from build123d import *

# Parameters (mm, degrees)
SKETCH_1_R      = 2
EXTRUDE_1_DEPTH = 3
EXTRUDE_2_DEPTH = 3
RIB_6_REACH     = 175.393
SKETCH_4_WALL_W = 365.010042788
SKETCH_4_WALL_H = 3
RIB_7_REACH     = 175.393
SKETCH_5_WALL_W = 365.010042788
SKETCH_5_WALL_H = 3
FILLET_1_R      = 2


with BuildPart() as part:
    # Эскиз1 → Бобышка-Вытянуть1 (new body)
    with BuildSketch(Plane(origin=(0, 0, 0), x_dir=(0, 0, -1), z_dir=(1, 0, 0))):
        with BuildLine():
            Line((0, 3), (0, 83))
            ThreePointArc((0, 83), (0.878679656, 85.121320344), (3, 86))
            Line((3, 86), (147, 86))
            ThreePointArc((147, 86), (149.121320344, 85.121320344), (150, 83))
            Line((150, 83), (150, 3))
            ThreePointArc((150, 3), (149.121320344, 0.878679656), (147, 0))
            Line((147, 0), (3, 0))
            ThreePointArc((3, 0), (0.878679656, 0.878679656), (0, 3))
        make_face()
        with Locations((6, 80)):
            Circle(SKETCH_1_R, mode=Mode.SUBTRACT)
        with Locations((144, 80)):
            Circle(SKETCH_1_R, mode=Mode.SUBTRACT)
        with Locations((120, 6)):
            Circle(SKETCH_1_R, mode=Mode.SUBTRACT)
        with Locations((6, 16)):
            Circle(SKETCH_1_R, mode=Mode.SUBTRACT)
        with BuildLine():
            Line((9, 74.803847577), (9, 21.196152423))
            ThreePointArc((9, 21.196152423), (11.196152423, 19), (12, 16))
            Line((12, 16), (12, 12))
            ThreePointArc((12, 12), (12.878679656, 9.878679656), (15, 9))
            Line((15, 9), (114.803847577, 9))
            ThreePointArc((114.803847577, 9), (120, 12), (125.196152423, 9))
            Line((125.196152423, 9), (138, 9))
            ThreePointArc((138, 9), (140.121320344, 9.878679656), (141, 12))
            Line((141, 12), (141, 74.803847577))
            ThreePointArc((141, 74.803847577), (139.757359313, 75.757359313), (138.803847577, 77))
            Line((138.803847577, 77), (11.196152423, 77))
            ThreePointArc((11.196152423, 77), (10.242640687, 75.757359313), (9, 74.803847577))
        make_face(mode=Mode.SUBTRACT)
    extrude(amount=EXTRUDE_1_DEPTH)

    # Эскиз2 → Бобышка-Вытянуть2 (add)
    with BuildSketch(Plane(origin=(0, 0, -50), x_dir=(-1, 0, 0), z_dir=(0, 0, -1))):
        with BuildLine():
            Line((0, 86), (-13, 86))
            Line((-13, 86), (-13, 68))
            Line((-13, 68), (-6, 68))
            ThreePointArc((-6, 68), (-4, 66), (-6, 64))
            Line((-6, 64), (-13, 64))
            Line((-13, 64), (-13, 22))
            Line((-13, 22), (-6, 22))
            ThreePointArc((-6, 22), (-4, 20), (-6, 18))
            Line((-6, 18), (-13, 18))
            Line((-13, 18), (-13, 0))
            Line((-13, 0), (0, 0))
            Line((0, 0), (0, 86))
        make_face()
    extrude(amount=EXTRUDE_2_DEPTH)

    # Эскиз4 wall → Ребро6 (add, up to next)
    with BuildSketch(Plane(origin=(7.056201664, 86, -60.025547367), x_dir=(-0.499999999996, 0, -0.866025403787), z_dir=(-0.866025403787, 0, 0.499999999996)), mode=Mode.PRIVATE) as rib_6_sk1:
        with Locations((0, 1.5)):
            Rectangle(SKETCH_4_WALL_W, SKETCH_4_WALL_H)
    rib_6_tool1 = extrude(rib_6_sk1.sketch, amount=RIB_6_REACH, mode=Mode.PRIVATE) - part.part
    add(rib_6_tool1.solids().sort_by_distance((7.056201664, 86, -60.025547367))[0])

    # Эскиз5 wall → Ребро7 (add, up to next)
    with BuildSketch(Plane(origin=(7.056201664, 0, -60.025547367), x_dir=(-0.499999999996, 0, -0.866025403787), z_dir=(0.866025403787, 0, -0.499999999996)), mode=Mode.PRIVATE) as rib_7_sk1:
        with Locations((0, 1.5)):
            Rectangle(SKETCH_5_WALL_W, SKETCH_5_WALL_H)
    rib_7_tool1 = extrude(rib_7_sk1.sketch, amount=-RIB_7_REACH, mode=Mode.PRIVATE) - part.part
    add(rib_7_tool1.solids().sort_by_distance((7.056201664, 0, -60.025547367))[0])

    # Скругление1
    fillet_1_edges = [part.edges().sort_by_distance(p)[0] for p in [
        (1.5, 77, -50),
        (1.5, 77, -53),
        (1.5, 9, -50),
        (1.5, 9, -53),
    ]]
    fillet(fillet_1_edges, radius=FILLET_1_R)


solid = part.part
Build history of the part. All positions in model axes, mm. A direction names the side the tool comes from. Coordinates: 2 decimals unless noted, no trailing zeros. Write each loop counter-clockwise with the first axis right and the second up, starting at its lowest first coordinate (ties: lowest second). Pieces come first, ordered by that corner, then holes.
(1) Cut at D-D on x = 9.5. List the corners of the cut face in (y, z).
(2) Mould opens along Z. For faces 1 (the flat face through (7.11, 84.48, -59.93)), 2 (the flat face through (9, 18, -51)), 3 (the flat face through (1, 9, -31)) say: pulls with the +Z half, pulls with the -Z half, needs draft (parallel to the pull), parting line crosses it, or undercut.
(3) Cut at A-A on y = 60.5. List the corners of the cut face in (x, z).
(4) Cut at C-C on y = 6. List the corners of the cut face in (x, z).
(5) 3-axis set-ups, long thin cutter, end or side, ignore diameter. For faces 4 (the flat face through (2, 0, -75)), 5 (the flat face through (7, 44, -53)), 6 (the flat face through (1, 9, -132)), 7 (the flat face through (10, 22, -51)), 8 (the flat face through (6, 3, -57)): which of +Z, -Z, +X, -X, +Y, -Y reach the whole face in a straight line?
(6) Cut at B-B on z = -99. List the corners of the cut face in (x, y).
(7) Drill centre lines: line 1 (Y direction, x = 1.25, z = -6); line 2 (Y direction, x = 1.3, z = -120); line 3 (Y direction, x = 3.5, z = -58). Where is each one in solid material? Low to high.
(8) Pin check, flat tips, straight feed: pin 1 Ø1.5 at (x, y) = (4.5, 60.5) entering from -Z; pin 2 Ø2.5 at (y, z) = (80, -144) entering from +X; pin 3 Ø6.5 at (x, y) = (9, 27) entering from +Z. Stop position of each tip, or through.
Working result:
1. outline: (0, -55.79) - (3, -55.79) - (3, -53) - (18, -53) - (18, -50) - (0, -50) - close; (22, -53) - (64, -53) - (64, -50) - (22, -50) - close; (68, -53) - (83, -53) - (83, -55.79) - (86, -55.79) - (86, -50) - (68, -50) - close
2. face 1: pulls with the -Z half
2. face 2: needs draft
2. face 3: undercut
3. outline: (0, -150) - (3, -150) - (3, -141) - (0, -141) - close; (0, -53) - (13, -53) - (13, -50) - (0, -50) - close; (0, -9) - (3, -9) - (3, 0) - (0, 0) - close
4. outline: (0, -150) - (3, -150) - (3, -122) - (0, -122) - close; (0, -118) - (3, -118) - (3, -53) - (13, -53) - (13, -50) - (3, -50) - (3, 0) - (0, 0) - close
5. face 4: +Z, -Z, +X, -X, -Y
5. face 5: +X
5. face 6: +X, -X
5. face 7: +Z, -Z, +X
5. face 8: -Z, +X
6. outline: (0, 0) - (3, 0) - (3, 9) - (0, 9) - close; (0, 77) - (3, 77) - (3, 86) - (0, 86) - close
7. line 1: y = 0 to 14, 18 to 78, 82 to 86
7. line 2: y = 0 to 4, 8 to 12, 77 to 86
7. line 3: y = 0 to 3, 83 to 86
8. pin 1: stops at z = -53
8. pin 2: passes through
8. pin 3: stops at z = -50
